```python
from build123d import *

# Parameters (mm, degrees)
F0_R     = 10
F1_DEPTH = 25
F2_DEPTH = 50
F3_SIZE  = 2
F4_DEPTH = 35
F5_SIZE  = 2


with BuildPart() as f1:
    # F0 (on Front) → F1 (new body)
    with BuildSketch(Plane.XZ):
        with BuildLine():
            ThreePointArc((2.083333, -24.913043), (18.399502, -16.92508), (25, 0))
            ThreePointArc((25, 0), (18.399502, 16.92508), (2.083333, 24.913043))
            ThreePointArc((2.083333, 24.913043), (-25, 0), (2.083333, -24.913043))
        make_face()
        Circle(F0_R, mode=Mode.SUBTRACT)
        with BuildLine():
            ThreePointArc((2.083333, 24.913043), (18.399502, 16.92508), (25, 0))
            ThreePointArc((25, 0), (18.399502, -16.92508), (2.083333, -24.913043))
            Line((2.083333, -24.913043), (91.458333, -17.43913))
            ThreePointArc((91.458333, -17.43913), (72.5, 0), (91.458333, 17.43913))
            Line((91.458333, 17.43913), (2.083333, 24.913043))
        make_face()
        with BuildLine():
            ThreePointArc((107.5, 0), (102.879651, 11.847556), (91.458333, 17.43913))
            ThreePointArc((91.458333, 17.43913), (72.5, 0), (91.458333, -17.43913))
            ThreePointArc((91.458333, -17.43913), (102.879651, -11.847556), (107.5, 0))
        make_face()
        with Locations((90, 0)):
            Circle(F0_R, mode=Mode.SUBTRACT)
    extrude(amount=F1_DEPTH)

    # F0 (on Front) → F2 (join)
    with BuildSketch(Plane.XZ):
        with BuildLine():
            ThreePointArc((2.083333, -24.913043), (18.399502, -16.92508), (25, 0))
            ThreePointArc((25, 0), (18.399502, 16.92508), (2.083333, 24.913043))
            ThreePointArc((2.083333, 24.913043), (-25, 0), (2.083333, -24.913043))
        make_face()
        Circle(F0_R, mode=Mode.SUBTRACT)
    extrude(amount=F2_DEPTH)

    # F3
    f3_edges = [f1.edges().sort_by_distance(p)[0] for p in [
        (-2.083333, -50, 24.913043),
        (-10, -50, 0),
        (80, -25, 0),
    ]]
    chamfer(f3_edges, length=F3_SIZE)

    # F0 (on Front) → F4 (join)
    with BuildSketch(Plane.XZ):
        with BuildLine():
            ThreePointArc((107.5, 0), (102.879651, 11.847556), (91.458333, 17.43913))
            ThreePointArc((91.458333, 17.43913), (72.5, 0), (91.458333, -17.43913))
            ThreePointArc((91.458333, -17.43913), (102.879651, -11.847556), (107.5, 0))
        make_face()
        with Locations((90, 0)):
            Circle(F0_R, mode=Mode.SUBTRACT)
    extrude(amount=F4_DEPTH)

    # F5
    f5_edges = [f1.edges().sort_by_distance(p)[0] for p in [
        (80, -35, 0),
    ]]
    chamfer(f5_edges, length=F5_SIZE)


solid = f1.part
```
Source: CAD feature listing. Evaluate the final solid. Frame: model axes, mm. Coordinates: 2 decimals unless noted, no trailing zeros. Loops run counter-clockwise (first coordinate to the right, second up) from the corner with the lowest first, then second, coordinate; pieces in that order, holes last. Notation, with made-up numbers: (-37.75, -11) -> (9.25, -11) arc R22 ccw to (9.25, 13) -> close; hole circle Ø1 at (67, 81.5). An arc over 180 degrees is marked (long way). One line per item, written item: value. Start each with the question number.
Q1. Line query: line 1 along X through (y, z) = (-31, 4.5); line 2 along X through (y, z) = (-20.5, 4.5); line 3 along X through (y, z) = (-12.5, -1.5). Output: solid intervals per line, ascending.
Q2. Section query D-D, the plane z = -1.5. Give the number of separate pieces and of enclosed holes in the cut face, and give its area (3 significant figures).
Q3. Contact query for flat-ended pins moving along their axis: P1, Ø3, axis at x = 16, y = -25.5, coming from the -Z side; P2, Ø6, axis at x = 76, z = -8.5, coming from the -Y side; P3, Ø12, axis at x = 93.5, y = -6.5, coming from the -Z side; P4, Ø16, axis at x = 90, z = 0, coming from the +Y side. Output: stop coordinate, or through.
Q4. Mould query, pull axis Z, two halves, no side actions, for faces 1 (the face through (-2.17, -23.66, -9.76)), 2 (the face through (46.15, -12.32, -21.23)), 3 (the face through (94, -35, 12)). Classes: pulls with the +Z half, pulls with the -Z half, needs draft (parallel to the pull), parting line crosses it, or undercut.
Q5. Section query C-C, the plane y = -20. Return the cut outline in (x, z), and give its area (3 significant figures).
Q6. Section query A-A, the plane y = -31. Return the cut outline in (x, z).
Q7. Section query B-B, the plane x = 0. Return the cut outline in (y, z), and give its area (3 significant figures).
Results:
1. line 1: -24.59 to -8.93, 8.93 to 24.59, 73.09 to 81.07, 98.93 to 106.91
1. line 2: -24.59 to -8.93, 8.93 to 81.07, 98.93 to 106.91
1. line 3: -24.95 to -9.89, 9.89 to 80.11, 99.89 to 107.44
2. separate pieces: 3
2. enclosed holes: 0
2. area: 3,210 mm^2
3. P1: z = -23.87
3. P2: y = -35
3. P3: z = -17.77
3. P4: through
4. face 1: undercut
4. face 2: pulls with the -Z half
4. face 3: needs draft
5. outline: (2.08, -24.91) -> (91.46, -17.44) arc R17.5 ccw to (91.46, 17.44) -> (2.08, 24.91) arc R25 ccw (long way) to start; hole circle Ø20 at (0, 0); hole circle Ø20 at (90, 0)
5. area: 4,670 mm^2
6. outline: (2.08, -24.91) arc R25 ccw to (25, 0) arc R25 ccw to (2.08, 24.91) arc R25 ccw (long way) to start; circle Ø35 at (90, 0); hole circle Ø20 at (0, 0); hole circle Ø20 at (90, 0)
7. outline: (-50, -23) -> (-48, -25) -> (0, -25) -> (0, -10) -> (-48, -10) -> (-50, -12) -> close; (-50, 12) -> (-48, 10) -> (0, 10) -> (0, 25) -> (-48, 25) -> (-50, 23) -> close
7. area: 1,490 mm^2
